The listing builds one solid part. Answer for the finished solid, in the listing's coordinates (mm). Give positions to 0.01 mm unless a question says otherwise; leave off trailing zeros. Loops run counter-clockwise (first coordinate to the right, second up) from the corner with the lowest first, then second, coordinate; pieces in that order, holes last. Notation, with made-up numbers: (60.5, 19.5) - (110.5, 19.5) arc R22 ccw to (110.5, 50.5) - close; hole circle Ø6 at (43.25, -26). An arc over 180 degrees is marked (long way). Answer in a Markdown table with one row per item. Add a question column.
```python
from build123d import *

# Parameters (mm, degrees)
SKETCH2_W            = 31
SKETCH2_H            = 45
BOSS_EXTRUDE1_DEPTH  = 5
M5_CLEARANCE_HOLE1_D = 5.5
FILLET1_R            = 5


with BuildPart() as part:
    # Sketch2 → Boss-Extrude1 (new body)
    with BuildSketch(Plane.XY):
        Polygon((-10, 30), (-10, 10), (10, 10), (10, -10), (-10, -10), (-10, -52), (67.5, -52), (67.5, 30), align=None)
        with BuildLine():
            Line((19, 26.5), (60, 26.5))
            ThreePointArc((60, 26.5), (62, 24.5), (60, 22.5))
            Line((60, 22.5), (19, 22.5))
            ThreePointArc((19, 22.5), (17, 24.5), (19, 26.5))
        make_face(mode=Mode.SUBTRACT)
        with BuildLine():
            Line((19, -42.5), (60, -42.5))
            ThreePointArc((60, -42.5), (62, -44.5), (60, -46.5))
            Line((60, -46.5), (19, -46.5))
            ThreePointArc((19, -46.5), (17, -44.5), (19, -42.5))
        make_face(mode=Mode.SUBTRACT)
        with Locations((39.5, -10)):
            Rectangle(SKETCH2_W, SKETCH2_H, mode=Mode.SUBTRACT)
    extrude(amount=BOSS_EXTRUDE1_DEPTH)

    # M5 Clearance Hole1 (through all)
    with Locations(Plane.XY.offset(5)):
        with Locations((0, 20), (0, -20)):
            Hole(M5_CLEARANCE_HOLE1_D / 2)

    # Fillet1
    fillet1_edges = [part.edges().sort_by_distance(p)[0] for p in [
        (67.5, 30, 2.5),
        (67.5, -52, 2.5),
        (-10, -52, 2.5),
        (-10, -10, 2.5),
        (10, -10, 2.5),
        (10, 10, 2.5),
        (-10, 10, 2.5),
        (-10, 30, 2.5),
    ]]
    fillet(fillet1_edges, radius=FILLET1_R)


solid = part.part
```
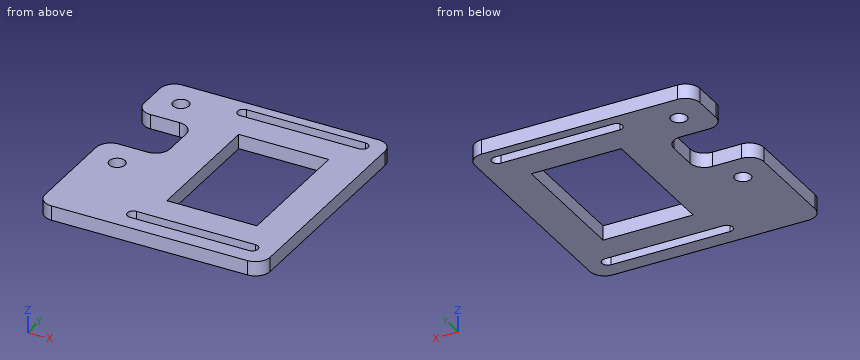
(1) A cutting plane is placed at D-D on y = -20. Determine the outline of the cut face in (x, z), plus the area to 3 significant figures.
(2) A cutting plane is placed at A-A on x = 30.5. Determine the outline of the cut face in (y, z), plus the area to 3 significant figures.
(3) A cutting plane is placed at C-C on y = 21.5. Determine the outline of the cut face in (x, z), plus the area to 3 significant figures.
(4) Given pin 1 Ø1.5 at (y, z) = (-0.5, 3) entering from -X; pin 2 Ø3.5 at (x, y) = (0, 20) entering from -Z, each flat-ended and moving along its own axis, determine where each tip first touches the part or whether it passes through.
(5) Find the intervals of material crossed by line 1 along Y through (x, z) = (0, 3.1); line 2 along Y through (x, z) = (36.5, 4.6); line 3 along X through (y, z) = (2, 4.3), in increasing order. Write a range as [from, to].
(6) A cutting plane is placed at B-B on z = 4. Give the number of separate pieces and of enclosed holes in the cut face, plus the area to 3 significant figures.
Evaluation:
| question | item | result |
|---|---|---|
| 1 | outline | (-10, 0) - (-2.75, 0) - (-2.75, 5) - (-10, 5) - close; (2.75, 0) - (24, 0) - (24, 5) - (2.75, 5) - close; (55, 0) - (67.5, 0) - (67.5, 5) - (55, 5) - close |
| 1 | area | 205 mm² |
| 2 | outline | (-52, 0) - (-46.5, 0) - (-46.5, 5) - (-52, 5) - close; (-42.5, 0) - (-32.5, 0) - (-32.5, 5) - (-42.5, 5) - close; (12.5, 0) - (22.5, 0) - (22.5, 5) - (12.5, 5) - close; (26.5, 0) - (30, 0) - (30, 5) - (26.5, 5) - close |
| 2 | area | 145 mm² |
| 3 | outline | (-10, 0) - (-2.3, 0) - (-2.3, 5) - (-10, 5) - close; (2.3, 0) - (67.5, 0) - (67.5, 5) - (2.3, 5) - close |
| 3 | area | 364 mm² |
| 4 | pin 1 | stops at x = 10 |
| 4 | pin 2 | passes through |
| 5 | line 1 | y = [-52, -22.75], [-17.25, -10], [10, 17.25], [22.75, 30] |
| 5 | line 2 | y = [-52, -46.5], [-42.5, -32.5], [12.5, 22.5], [26.5, 30] |
| 5 | line 3 | x = [10, 24], [55, 67.5] |
| 6 | separate pieces | 1 |
| 6 | enclosed holes | 5 |
| 6 | area | 4,140 mm² |
